CAD build for the part. Positions are in the model's coordinates, mm. Coordinates: 2 decimals unless noted, no trailing zeros. Loops run counter-clockwise (first coordinate to the right, second up) from the corner with the lowest first, then second, coordinate; pieces in that order, holes last. Notation, with made-up numbers: (53, 82.25) -> (57, 82.25) arc R21 cw to (57, 97.25) -> close; hole circle Ø1 at (39, 45). An arc over 180 degrees is marked (long way). Write each question's results on one line, items separated by ' | '.
```python
from build123d import *

# Parameters (mm, degrees)
BOSS_EXTRUDE1_DEPTH         = 90
TAP_DRILL_FOR_M5X0_8_TAP1_D = 4.2


with BuildPart() as part:
    # Sketch1 → Boss-Extrude1 (new body)
    with BuildSketch(Plane.XY):
        with BuildLine():
            Line((-31.734248061, 1), (-17.721808598, 1))
            ThreePointArc((-17.721808598, 1), (0, 17.75), (17.721808598, 1))
            Line((17.721808598, 1), (31.734248061, 1))
            ThreePointArc((31.734248061, 1), (0, 31.75), (-31.734248061, 1))
        make_face()
    extrude(amount=BOSS_EXTRUDE1_DEPTH)

    # Tap Drill for M5x0.8 Tap1 (through all)
    with Locations(Plane(origin=(-24.72802833, 1, 80), x_dir=(0, 0, -1), z_dir=(0, -1, 0))):
        with Locations((0, 0), (70, 0), (0, 49.45605666), (70, 49.45605666)):
            Hole(TAP_DRILL_FOR_M5X0_8_TAP1_D / 2)


solid = part.part
```
Q1. Wall check: L1, parallel to Z at x = 26, y = 9; L2, parallel to X at y = 10.25, z = 10; L3, parallel to Y at x = -1, z = 6.5. Give the ranges that are in metal, low to high. Write a range as from..to.
Results are:
L1: 0..8.33, 11.67..78.33, 81.67..90 | L2: -30.05..-26.83, -22.63..-14.49, 14.49..22.63, 26.83..30.05 | L3: 17.72..31.73
Q2. Pull direction Z, two halves, no side cores. Call faces 1 (the cylindrical face through (22.68, 11.78, 79.54)), 2 (the flat face through (0, 20, 90)), 3 (the flat face through (25, 1, 44)): +Z half, -Z half, draft (parallel to the pull), parting line (faces both ways), or undercut.
Results are:
face 1: undercut | face 2: +Z half | face 3: draft
Q3. Cut at A-A on y = 9. Write the cut outline in (x, z).
Results are:
outline: (-30.45, 0) -> (-15.3, 0) -> (-15.3, 90) -> (-30.45, 90) -> close; (15.3, 0) -> (30.45, 0) -> (30.45, 90) -> (15.3, 90) -> close; hole circle Ø4.2 at (-24.73, 10); hole circle Ø4.2 at (-24.73, 80); hole circle Ø4.2 at (24.73, 10); hole circle Ø4.2 at (24.73, 80)
Q4. Cut at B-B on z = 10. Write the cut outline in (x, y), and give its area (3 significant figures).
Results are:
outline: (-31.73, 1) -> (-26.83, 1) -> (-26.83, 16.98) arc R31.75 ccw to start; (-22.63, 1) -> (-17.72, 1) arc R17.75 cw to (17.72, 1) -> (22.63, 1) -> (22.63, 22.27) arc R31.75 ccw to (-22.63, 22.27) -> close; (26.83, 1) -> (31.73, 1) arc R31.75 ccw to (26.83, 16.98) -> close | area: 902 mm^2
Q5. Cut at C-C on x = 0. Write the cut outline in (y, z), and give its area (3 significant figures).
Results are:
outline: (17.75, 0) -> (31.75, 0) -> (31.75, 90) -> (17.75, 90) -> close | area: 1,260 mm^2
Q6. Drop flat-ended pins along their axis: pin 1 (12 mm diameter, centred on x = -24, z = 43, fed in from +Y); pin 2 (3 mm diameter, centred on y = 14, z = 75, fed in from -X); pin 3 (4 mm diameter, centred on y = 7, z = 46, fed in from +X). Give the stop position or say it passes through.
Results are:
pin 1: y = 26.15 | pin 2: x = -29.19 | pin 3: x = 31.35
